```python
from build123d import *

# Parameters (mm, degrees)
SKETCH1_W                                            = 100
SKETCH1_H                                            = 124.5
BOSS_EXTRUDE1_DEPTH                                  = 505
M8_TAPPED_HOLE1_D                                    = 6.8
M8_TAPPED_HOLE1_DEPTH                                = 22.25
M8_TAPPED_HOLE1_TIP                                  = 2.042926105
CBORE_FOR_M12_HEX_SOCKET_HEAD_CAP_SCREW1_D           = 13
CBORE_FOR_M12_HEX_SOCKET_HEAD_CAP_SCREW1_CBORE_D     = 20
CBORE_FOR_M12_HEX_SOCKET_HEAD_CAP_SCREW1_CBORE_DEPTH = 12.6
LPATTERN1_COUNT                                      = 12
LPATTERN1_PITCH                                      = 80


with BuildPart() as part:
    # Sketch1 → Boss-Extrude1 (new, symmetric)
    with BuildSketch(Plane(origin=(0, 0, 0), x_dir=(0, 0, -1), z_dir=(1, 0, 0))):
        Rectangle(SKETCH1_W, SKETCH1_H)
    extrude(amount=BOSS_EXTRUDE1_DEPTH, both=True)

    # M8 Tapped Hole1
    with Locations(Plane(origin=(0, 62.25, 0), x_dir=(1, 0, 0), z_dir=(0, 1, 0))):
        with Locations((480, 30), (480, -30), (400, 30), (400, -30), (320, 30), (320, -30), (240, -30), (240, 30), (160, 30), (160, -30), (80, 30), (80, -30), (0, -30), (0, 30), (-80, -30), (-80, 30), (-160, -30), (-160, 30), (-240, -30), (-240, 30), (-320, -30), (-320, 30), (-400, -30), (-400, 30), (-480, 30), (-480, -30)):
            Hole(M8_TAPPED_HOLE1_D / 2, depth=M8_TAPPED_HOLE1_DEPTH)
            with Locations((0, 0, -(M8_TAPPED_HOLE1_DEPTH + M8_TAPPED_HOLE1_TIP / 2))):  # 118° drill point
                Cone(0, M8_TAPPED_HOLE1_D / 2, M8_TAPPED_HOLE1_TIP, mode=Mode.SUBTRACT)

    # CBORE for M12 Hex Socket Head Cap Screw1 (through all)
    with Locations(Plane(origin=(0, 62.25, 0), x_dir=(1, 0, 0), z_dir=(0, 1, 0))):
        with Locations((440, 0)):
            cbore_for_m12_hex_socket_head_cap_screw1 = CounterBoreHole(CBORE_FOR_M12_HEX_SOCKET_HEAD_CAP_SCREW1_D / 2, CBORE_FOR_M12_HEX_SOCKET_HEAD_CAP_SCREW1_CBORE_D / 2, CBORE_FOR_M12_HEX_SOCKET_HEAD_CAP_SCREW1_CBORE_DEPTH)

    # LPattern1: CBORE for M12 Hex Socket Head Cap Screw1 ×12
    with Locations(*[(-i * LPATTERN1_PITCH, 0, 0) for i in range(1, LPATTERN1_COUNT)]):
        add(cbore_for_m12_hex_socket_head_cap_screw1, mode=Mode.SUBTRACT)


solid = part.part
```
Build history of the part. All positions in model axes, mm. A direction names the side the tool comes from. Round coordinates to 2 decimals unless told otherwise and drop trailing zeros.
1) 3-axis set-ups, long thin cutter, end or side, ignore diameter. For faces 5 (the cylindrical face through (449.54, 56.04, -3)), 6 (the flat face through (7, 62.25, 1)): which of +Z, -Z, +X, -X, +Y, -Y reach the whole face in a straight line?
2) Mould opens along X. For faces 1 (the flat face through (7, -1, -50)), 2 (the cylindrical face through (-190.763, 56.038, 3.83)), 3 (the flat face through (505, 1, 1)), 4 (the flat face through (440, 49.65, 7)) say: +X half, -X half, draft (parallel to the pull), parting line (faces both ways), or undercut.
3) Band-saw the part on A-A, the plane y = -19. Give the number of separate pieces and of enclosed holes in the cut face, and give its area (3 significant figures).
4) Drill centre lines: probe 1 along Z at (x, y) = (-400, 46.25); probe 2 along Z at (x, y) = (-360, 27); probe 3 along Z at (x, y) = (-362, -43.5). Where is each one in solid material? Low to high.
5) Pin check, flat tips, straight feed: pin 1 (23 mm diameter, centred on x = -360, z = 0, fed in from +Y); pin 2 (4 mm diameter, centred on x = 160, z = 30, fed in from +Y); pin 3 (16 mm diameter, centred on x = 360, z = 0, fed in from +Y); pin 4 (10.5 mm diameter, centred on x = 360, z = 0, fed in from +Y). Stop position of each tip, or through.
Ans:
1. face 5: +Y
1. face 6: +Z, -Z, +X, -X, +Y
2. face 1: draft
2. face 2: undercut
2. face 3: +X half
2. face 4: undercut
3. separate pieces: 1
3. enclosed holes: 12
3. area: 99,400 mm2
4. probe 1: z = -50 to -33.4, -26.6 to 26.6, 33.4 to 50
4. probe 2: z = -50 to -6.5, 6.5 to 50
4. probe 3: z = -50 to -6.18, 6.18 to 50
5. pin 1: stops at y = 62.25
5. pin 2: stops at y = 39.16
5. pin 3: stops at y = 49.65
5. pin 4: passes through
